Autodesk Fusion 360 part; units mm, degrees
sketch "T_v1_Arm_5_Inch_Shorty_6mm_or_5mm_4x" plane through (0, 0, 0) normal (0, 0, 1) x (1, 0, 0)
  arc A0 (-225.6533, 220.9552) -> (-220.6279, 220.4722) centre (-222.8873, 223.3495) ccw
  arc A1 (-230.3335, 140.9887) -> (-229.5344, 133.9506) centre (-220.257, 138.5683) ccw
  arc A2 (-217.3945, 140.1231) -> (-217.1516, 139.4711) centre (-212.5989, 141.5382) ccw
  line L0 (-215.5389, 136.8403) -> (-226.8186, 127.742)
  arc A3 (-215.5389, 136.8403) -> (-214.3199, 135.521) centre (-209.8871, 140.8396) ccw
  arc A4 (-215.7785, 202.7474) -> (-216.6488, 201.3936) centre (-212.0626, 199.402) ccw
  arc A5 (-215.0172, 213.5689) -> (-220.6279, 220.4722) centre (-217.8805, 216.9734) ccw
  arc A6 (-220.2406, 159.5651) -> (-217.3945, 140.1231) centre (-150.6263, 159.8267) ccw
  arc A7 (-215.7785, 202.7474) -> (-215.5657, 208.4451) centre (-219.0846, 205.7238) ccw
  circle A8 centre (-217.8805, 216.9734) radius 1.5
  arc A9 (-228.9289, 130.3582) -> (-229.2844, 133.4743) centre (-231.6499, 131.6261) ccw
  circle A10 centre (-224.0861, 140.4692) radius 1.45
  circle A11 centre (-218.5249, 129.3701) radius 1.45
  arc A12 (-216.6488, 201.3936) -> (-220.3306, 183.5032) centre (-175.8354, 183.6704) ccw
  arc A13 (-225.6533, 220.9552) -> (-232.9473, 215.8914) centre (-229.1297, 218.1776) ccw
  arc A14 (-229.5344, 133.9506) -> (-229.2844, 133.4743) centre (-228.5434, 134.167) ccw
  circle A15 centre (-219.0847, 205.7238) radius 1.5
  arc A16 (-211.6169, 132.1699) -> (-210.5855, 130.6992) centre (-205.2604, 135.5308) ccw
  arc A17 (-217.1516, 139.4711) -> (-215.5389, 136.8403) centre (-205.7671, 144.6403) ccw
  line L1 (-221.8653, 121.601) -> (-228.9289, 130.3582)
  circle A18 centre (-224.0878, 211.9497) radius 3.5
  circle A19 centre (-218.5249, 129.3701) radius 1.45
  arc A20 (-228.2024, 185.7996) -> (-232.5238, 214.992) centre (-304.8727, 189.366) ccw
  line L2 (-220.2406, 159.5651) -> (-220.3306, 183.5032)
  circle A21 centre (-229.1297, 218.1776) radius 1.5
  arc A22 (-232.5238, 214.992) -> (-232.9473, 215.8914) centre (-237.2369, 213.3226) ccw
  arc A23 (-211.6169, 132.1699) -> (-214.3199, 135.521) centre (-218.6052, 129.2988) ccw
  line L3 (-210.5855, 130.6992) -> (-221.8653, 121.601)
  arc A24 (-215.0172, 213.5689) -> (-215.5657, 208.4451) centre (-212.6223, 210.7213) ccw
  arc A25 (-228.2024, 185.7996) -> (-230.2645, 141.4764) centre (17543.3039, -663.1993) ccw
  arc A26 (-230.3335, 140.9887) -> (-230.2645, 141.4764) centre (-232.8519, 141.5936) ccw
extrude "Extrude1" add sketch "T_v1_Arm_5_Inch_Shorty_6mm_or_5mm_4x" against normal blind 5.5 makes body 1
extrude "Extrude2" cut sketch "T_v1_Arm_5_Inch_Shorty_6mm_or_5mm_4x" against normal blind 2.75 contours L0 A3 A16 L1 A23 L3 bodies 1
extrude "Extrude3" add sketch "T_v1_Arm_5_Inch_Shorty_6mm_or_5mm_4x" against normal blind 6 separate body makes body 2
extrude "Extrude4" cut sketch "T_v1_Arm_5_Inch_Shorty_6mm_or_5mm_4x" against normal blind 3 contours L0 A3 A16 L1 A23 L3 bodies 2
hidden bodies 1
CAD build for the part. Positions are in the model's coordinates, mm. A direction names the side the tool comes from. Coordinates: 2 decimals unless noted, no trailing zeros. Order: outer loops, then holes, each group sorted by start corner. A loop starts at its lowest first (then second) coordinate and runs counter-clockwise, first axis right, second up. Notation, with made-up numbers: M -2,-28 L 5,-28 A11 cw 5,-12 Z; hole C -4.75,-16 d3. An arc over 180 degrees is marked long. Write each question's results on one line, items separated by ' | '. Start each with the question number.
Q1. Pull direction Y, two halves, no side cores. Call faces 5 (the flat face through (-221.1, 132.355, -1.479)), 6 (the cylindrical face through (-231.59, 221.885, -2.958)), 7 (the cylindrical face through (-228.665, 131.943, -2.958)): +Y half, -Y half, draft (parallel to the pull), parting line (faces both ways), or undercut.
Q2. Cut at A-A (z = -4.95). Count the separate pieces of the cut face and the enclosed holes in it, then the cut area to 3 significant figures.
Q3. Cut at C-C (y = 154). List the corners of the cut face in (x, z).
Q4. Drill centre lines: probe 1 along Y at (x, z) = (-216, -2.7); probe 2 along Y at (x, z) = (-225.25, -4.3); probe 3 along Y at (x, z) = (-222, -3.45). Where is each one in solid material? Low to high. Write a range as from..to.
Q5. Flat gauge pins, fed straight in: P1, Ø1.5, axis at y = 177.5, z = -3, coming from the +X side; P2, Ø1, axis at y = 195, z = -3.5, coming from the +X side; P3, Ø7.5, axis at x = -218.5, y = 126.5, coming from the +Z side; P4, Ø4, axis at x = -217.88, y = 216.97, coming from the +Z side. Where does each tip first touch, or does it go through?
Q6. Which spindle directions (+Z, -Z, +X, -X, +Y, -Y) get a long thin tool onto all of the face, cutting with end or side? Do faces 1 (the flat face through (-219, 131, -3)), 2 (the cylindrical face through (-216.438, 138.124, -2.958)), 3 (the cylindrical face through (-229.233, 163.949, -2.958)), 4 (the flat face through (-216.15, 126.21, -4.48)). Say none if no direction does.
Q7. Cut at B-B (y = 138). List the corners of the cut face in (x, z).
Found:
1) face 5: -Y half | face 6: parting line | face 7: undercut
2) separate pieces: 1 | enclosed holes: 6 | area: 1,060 mm²
3) outline: M -229.69,-6 L -220,-6 L -220,0 L -229.69,0 Z
4) probe 1: 136.47..137.46, 202.48..209.16, 212.28..221 | probe 2: 125.8..139.6, 141.33..208.65, 215.25..220.56 | probe 3: 121.77..209.14, 214.76..219.8
5) P1: x = -220.31 | P2: x = -218.73 | P3: z = -3 | P4: z = 0
6) face 1: +Z, +X, -Y | face 2: +Z, -Z, +X | face 3: +Z, -Z, -X | face 4: +Z, -Z, +X, -Y
7) outline: M -230.6,-6 L -216.36,-6 L -216.36,0 L -230.6,0 Z
